For this review, take the finished solid that the model builds, in its own axes (mm). A direction names the side the tool comes from. Give positions to 0.01 mm unless a question says otherwise; leave off trailing zeros. Loops run counter-clockwise (first coordinate to the right, second up) from the corner with the lowest first, then second, coordinate; pieces in that order, holes last. Notation, with made-up numbers: (14, 87) -> (67, 87) arc R18 cw to (67, 94) -> close; hole circle Ø8 at (36, 12.5). An arc over 180 degrees is marked (long way). Answer as CSV lines item,"result". Start each with the question number.
Item 1: Add section C-C on z = 2.75. State the section outline as (x, y) points.
Item 2: The part is to be moulded in two halves that separate along Y. For faces 4 (the face through (12.522, -3.909, 2.433)), 5 (the face through (12, -6.35, 3)), 6 (the face through (13.69, -3.13, 1.12)), say which applies: +Y half, -Y half, draft (parallel to the pull), parting line (faces both ways), or undercut.
Item 3: For L1, parallel to X at y = -4, z = 1.25; L2, parallel to Z at x = 10, y = -2; L3, parallel to Y at x = 2.5, z = 5.25, list the stretches that pass through material, from the lowest coordinate up. Write a range as from..to.
Item 4: Add section B-B on x = 12.7. State the section outline as (y, z) points (3 decimals).
Item 5: Clearance check with flat-ended pins moving along their axes: P1, Ø3, axis at y = -5.5, z = 3, coming from the -X side; P2, Ø1.6, axis at y = -3, z = 4.5, coming from the +X side; P3, Ø1, axis at y = -5.5, z = 4, coming from the +X side; P4, Ø3, axis at x = 27.5, y = -2, coming from the +Z side. State where each tip first meets the part, or that it passes through.
Item 6: Add section A-A on y = -1.25. State the section outline as (x, z) points, plus the area to 3 significant figures.
Item 7: Add section D-D on x = 29. State the section outline as (y, z) points, plus the area to 3 significant figures.
Item 8: Machinability: for faces 1 (the face through (13, -3, 6.35)), 2 (the face through (27, -3, 1)), 3 (the face through (0, -5, 3)), which of the approach directions +Z, -Z, +X, -X, +Y, -Y give a long, thin tool a straight path to every point of the face, cutting with its end or side? Answer none if there is none.
```python
from build123d import *

# Parameters (mm, degrees)
SKETCH1_W             = 6.35
SKETCH1_H             = 6.35
SKETCH1_R             = 1.4732
BOSS_EXTRUDE1_DEPTH   = 1
BOSS_EXTRUDE1_2_DEPTH = 1
SKETCH1_3_W           = 25.4
SKETCH1_3_H           = 6.35
BOSS_EXTRUDE2_DEPTH   = 6.35
SKETCH2_R             = 1.591
CUT_EXTRUDE1_DEPTH    = 25.4
SKETCH3_R             = 1
CUT_EXTRUDE2_DEPTH    = 6.35


with BuildPart() as part:
    # Sketch1 → Boss-Extrude1 (new body)
    with BuildSketch(Plane.XY):
        with Locations((-3.175, -3.175)):
            Rectangle(SKETCH1_W, SKETCH1_H)
        with Locations((-3.275, -3.175)):
            Circle(SKETCH1_R, mode=Mode.SUBTRACT)
    extrude(amount=BOSS_EXTRUDE1_DEPTH)



with BuildPart() as body_2:
    # Sketch1 → Boss-Extrude1 2 (new body)
    with BuildSketch(Plane.XY):
        with Locations((28.575, -3.175)):
            Rectangle(SKETCH1_W, SKETCH1_H)
        with Locations((28.675, -3.175)):
            Circle(SKETCH1_R, mode=Mode.SUBTRACT)
    extrude(amount=BOSS_EXTRUDE1_2_DEPTH)


with BuildPart() as part_1:
    add(part.part)

    add(body_2.part)  # Boss-Extrude2 merges body 2
    # Sketch1<3> → Boss-Extrude2 (add)
    with BuildSketch(Plane.XY):
        with Locations((12.7, -3.175)):
            Rectangle(SKETCH1_3_W, SKETCH1_3_H)
    extrude(amount=BOSS_EXTRUDE2_DEPTH)

    # Sketch2 → Cut-Extrude1 (cut)
    with BuildSketch(Plane.ZY):
        with Locations(Location((3.8448, -3.175, 0), (0, 0, 270))):
            Circle(SKETCH2_R)
    extrude(amount=-CUT_EXTRUDE1_DEPTH, mode=Mode.SUBTRACT)

    # Sketch3 → Cut-Extrude2 (cut)
    with BuildSketch(Plane(origin=(0, 0, 0), x_dir=(1, 0, 0), z_dir=(0, 1, 0))):
        with Locations(Location((12.7, -1.25, 0), (0, 0, 270))):
            Circle(SKETCH3_R)
    extrude(amount=-CUT_EXTRUDE2_DEPTH, mode=Mode.SUBTRACT)


solid = part_1.part
```
Computed values:
1,outline,"(0, -6.35) -> (25.4, -6.35) -> (25.4, -4.33) -> (0, -4.33) -> close; (0, -2.02) -> (25.4, -2.02) -> (25.4, 0) -> (0, 0) -> close"
2,face 4,"undercut"
2,face 5,"-Y half"
2,face 6,"draft"
3,L1,"0..11.7, 13.7..25.4"
3,L2,"0..2.77, 4.92..6.35"
3,L3,"-6.35..-3.92, -2.43..0"
4,outline,"(-6.35, 0) -> (0, 0) -> (0, 0.25) -> (-6.35, 0.25) -> close; (-6.35, 2.25) -> (0, 2.25) -> (0, 6.35) -> (-6.35, 6.35) -> close; hole circle Ø3.182 at (-3.175, 3.845)"
5,P1,"x = 0"
5,P2,"through"
5,P3,"x = 25.4"
5,P4,"z = 1"
6,outline,"(-6.35, 0) -> (31.75, 0) -> (31.75, 1) -> (25.4, 1) -> (25.4, 6.35) -> (0, 6.35) -> (0, 1) -> (-6.35, 1) -> close; hole circle Ø2 at (12.7, 1.25)"
6,area,"171 mm²"
7,outline,"(-6.35, 0) -> (-4.61, 0) -> (-4.61, 1) -> (-6.35, 1) -> close; (-1.74, 0) -> (0, 0) -> (0, 1) -> (-1.74, 1) -> close"
7,area,"3.48 mm²"
8,face 1,"+Z, +X, -X, +Y, -Y"
8,face 2,"+Z, +X, +Y, -Y"
8,face 3,"+Z, -X, +Y, -Y"
